Design review of the part built by this model. Coordinates are the model's own, in mm. Face numbers are marked on the shaded views. A direction names the side the tool comes from. Coordinates: 2 decimals unless noted, no trailing zeros. Loops run counter-clockwise (first coordinate to the right, second up) from the corner with the lowest first, then second, coordinate; pieces in that order, holes last. Notation, with made-up numbers: (15, 54.5) -> (28, 54.5) arc R12 ccw to (28, 67.5) -> close; hole circle Ø6 at (-4.5, 72.25). An arc over 180 degrees is marked (long way). Use a Markdown table: item, result. Add a question column.
Q1. For the marked faces 5 and 6, list the 3-axis set-ups (+Z, -Z, +X, -X, +Y, -Y) from which the entire face can be reached by the end or side of a thin tool; tool diameter is ignored.
Q2. Take a section at B-B on y = 0. Write out the cut boundary in (x, z).
Q3. Clearance check with flat-ended pins moving along their axes: pin 1 Ø1.8 at (x, z) = (-7, -0.5) entering from +Y; pin 2 Ø2 at (x, z) = (-10, 0) entering from +Y; pin 3 Ø4.5 at (x, z) = (-10, 0) entering from +Y; pin 4 Ø3 at (x, z) = (-6, 6) entering from +Y. State where each tip first meets the part, or that it passes through.
Q4. Take a section at C-C on x = -14.5. Write out the cut boundary in (y, z).
Q5. Take a section at A-A on z = 0. Count the separate pieces of the cut face and the enclosed holes in it, plus the area to 3 significant figures.
Q6. Take a section at D-D on x = -2.5. Write out the cut boundary in (y, z), plus the area to 3 significant figures.
Q7. For probe 1 along X at (y, z) = (4.7, 0); probe 2 along Y at (x, z) = (-7.5, -1.25); probe 3 along Y at (x, z) = (-8.75, -1.75), list the stretches that pass through material, from the lowest coordinate up.
Q8. Draft analysis for pull direction Z (two halves, no side actions). For the marked faces 1, 2, 3 and 4, state which applies: pulls with the +Z half, pulls with the -Z half, needs draft (parallel to the pull), parting line crosses it, or undercut.
from build123d import *

# Parameters (mm, degrees)
SKETCH_2_R          = 1.75
CUT_EXTRUDE_5_DEPTH = 27.229754097
CUT_EXTRUDE_START   = 12
SKETCH_2_4_R        = 3
CUT_EXTRUDE_6_DEPTH = 2
SKETCH_4_W          = 6
SKETCH_4_H          = 3
CUT_EXTRUDE_7_DEPTH = 15
FILLET_1_R          = 2


with BuildPart() as part:
    # Sketch 1 → Revolve 1 (revolve)
    with BuildSketch(Plane.XY, mode=Mode.PRIVATE) as revolve_1_sk:
        Polygon((-15, 3), (0, 3), (0, 4.5), (-4, 4.5), (-4, 12), (-20, 12), (-20, 0), (-15, 0), align=None)
    revolve(revolve_1_sk.sketch.rotate(Axis((-12.015902685, 0, 0), (1, 0, 0)), 90), axis=Axis((-12.015902685, 0, 0), (1, 0, 0)))

    # Sketch 2 → Cut-Extrude 5 (cut, through all)
    with BuildSketch(Plane(origin=(0, 0, 0), x_dir=(1, 0, 0), z_dir=(0, 1, 0))):
        with Locations(Location((-10, 0, 0), (0, 0, 90))):
            Circle(SKETCH_2_R)
    extrude(amount=CUT_EXTRUDE_5_DEPTH, mode=Mode.SUBTRACT)

    # Sketch 2_4 → Cut-Extrude 6 (cut)
    with BuildSketch(Plane(origin=(0, 0, 0), x_dir=(1, 0, 0), z_dir=(0, 1, 0)).offset(CUT_EXTRUDE_START)):
        with Locations(Location((-10, 0, 0), (0, 0, 270))):
            Circle(SKETCH_2_4_R)
    extrude(amount=-CUT_EXTRUDE_6_DEPTH, mode=Mode.SUBTRACT)

    # Sketch 4 → Cut-Extrude 7 (cut)
    with BuildSketch(Plane(origin=(0, 0, 0), x_dir=(0, 0, -1), z_dir=(1, 0, 0))):
        with Locations((0, 7)):
            Rectangle(SKETCH_4_W, SKETCH_4_H)
    extrude(amount=-CUT_EXTRUDE_7_DEPTH, mode=Mode.SUBTRACT)

    # Fillet 1
    fillet_1_edges = [part.edges().sort_by_distance(p)[0] for p in [
        (-20, 0, -12),
        (-4, 0, -12),
    ]]
    fillet(fillet_1_edges, radius=FILLET_1_R)


solid = part.part
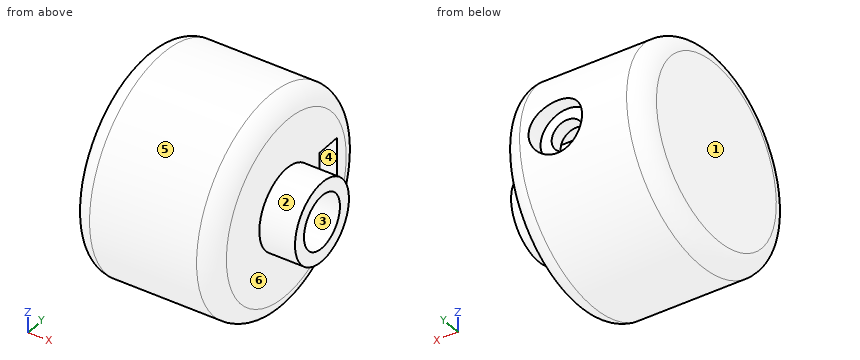
Answer list:
| question | item | result |
|---|---|---|
| 1 | face 5 | +X, -X |
| 1 | face 6 | +X |
| 2 | outline | (-20, -10) arc R2 ccw to (-18, -12) -> (-6, -12) arc R2 ccw to (-4, -10) -> (-4, -4.5) -> (0, -4.5) -> (0, -3) -> (-15, -3) -> (-15, 3) -> (0, 3) -> (0, 4.5) -> (-4, 4.5) -> (-4, 10) arc R2 ccw to (-6, 12) -> (-18, 12) arc R2 ccw to (-20, 10) -> close |
| 3 | pin 1 | y = 12 |
| 3 | pin 2 | y = -2.83 |
| 3 | pin 3 | y = 10 |
| 3 | pin 4 | y = 11.12 |
| 4 | outline | circle Ø24 at (0, 0); hole circle Ø6 at (0, 0); hole (5.5, -3) -> (8.5, -3) -> (8.5, 3) -> (5.5, 3) -> close |
| 5 | separate pieces | 3 |
| 5 | enclosed holes | 0 |
| 5 | area | 268 mm² |
| 6 | outline | circle Ø9 at (0, 0); hole circle Ø6 at (0, 0) |
| 6 | area | 35.3 mm² |
| 7 | probe 1 | -20 to -11.75, -8.25 to -4 |
| 7 | probe 2 | -11.93 to -2.73, 2.73 to 5.5, 8.5 to 10 |
| 7 | probe 3 | -11.87 to -2.44, 2.44 to 5.5, 8.5 to 10 |
| 8 | face 1 | needs draft |
| 8 | face 2 | parting line crosses it |
| 8 | face 3 | undercut |
| 8 | face 4 | undercut |
